Geometry: see drawing. Coordinates: mm, zero at the bounding-box minimum. A direction names the side the tool comes from. Coordinates: 2 decimals unless noted, no trailing zeros. Order: outer loops, then holes, each group sorted by start corner. A loop starts at its lowest first (then second) coordinate and runs counter-clockwise, first axis right, second up. Notation, with made-up numbers: M -21.5,-7 L 16.5,-7 A21 ccw 16.5,29 Z; hole C 3.5,51 d4. An arc over 180 degrees is marked long. Answer in a Markdown table with one row per item.
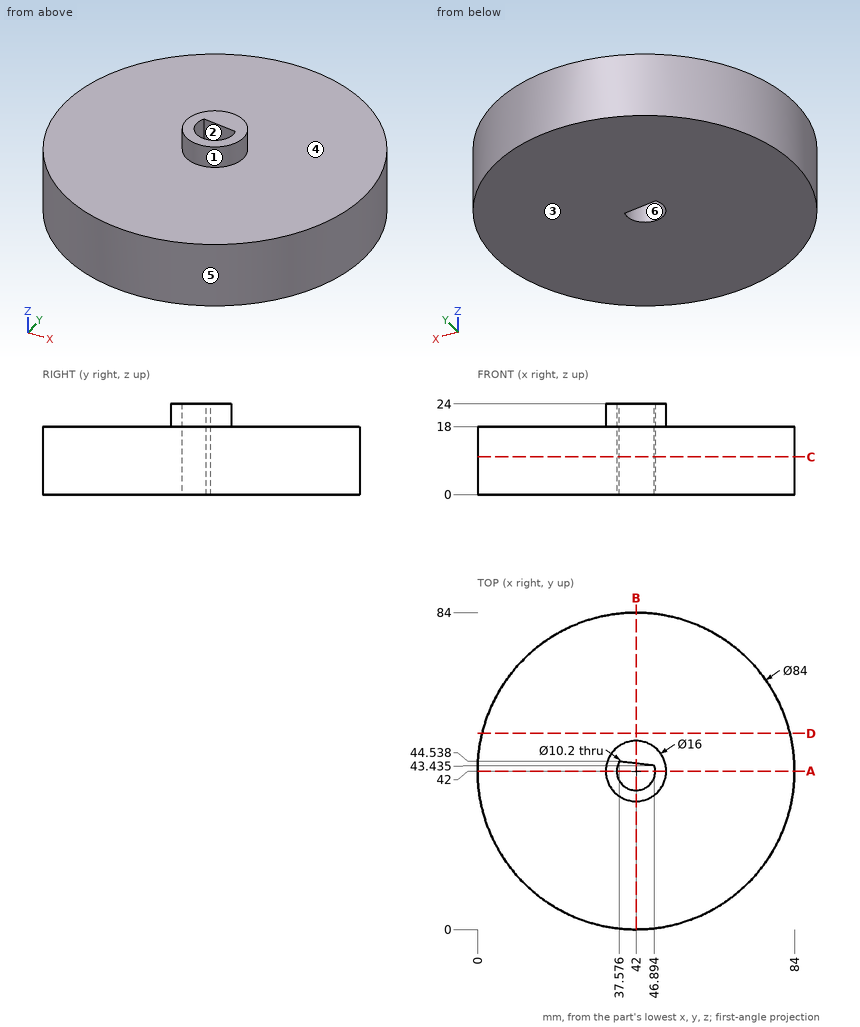
1) Cut plane D-D, the plane y = 52. Output: boundary loops of the cut face in (x, z).
Resolved:
| item | result |
|---|---|
| outline | M 1.21,0 L 82.79,0 L 82.79,18 L 1.21,18 Z |
2) Reachability of the marked faces 1, 2 and 3 from +Z, -Z, +X, -X, +Y, -Y: full face, straight path, thin tool, end or side. Return the list, or none.
Resolved:
| item | result |
|---|---|
| face 1 | +Z |
| face 2 | +Z, -Z |
| face 3 | -Z, +X, -X, +Y, -Y |
3) Contact query for flat-ended pins moving along their axis: pin 1 (5 mm diameter, centred on y = 17.5, z = 8.5, fed in from -X); pin 2 (3 mm diameter, centred on x = 30.5, y = 72.5, fed in from +Z); pin 3 (1.5 mm diameter, centred on x = 61, z = 20.5, fed in from +Y) (1 decimal); pin 4 (8 mm diameter, centred on y = 73, z = 13.5, fed in from -X). Output: stop coordinate, or through.
Resolved:
| item | result |
|---|---|
| pin 1 | stops at x = 6.22 |
| pin 2 | stops at z = 18 |
| pin 3 | passes through |
| pin 4 | stops at x = 9.83 |
4) Material intervals for probe 1 along X at (y, z) = (42, 15.25); probe 2 along Z at (x, y) = (15.5, 64); probe 3 along Y at (x, z) = (42, 12.5) (1 decimal), sorted ascending.
Resolved:
| item | result |
|---|---|
| probe 1 | x = 0 to 36.9, 47.1 to 84 |
| probe 2 | z = 0 to 18 |
| probe 3 | y = 0 to 36.9, 44 to 84 |
5) Cut plane A-A, the plane y = 42. Output: boundary loops of the cut face in (x, z).
Resolved:
| item | result |
|---|---|
| outline | M 0,0 L 36.9,0 L 36.9,24 L 34,24 L 34,18 L 0,18 Z; M 47.1,0 L 84,0 L 84,18 L 50,18 L 50,24 L 47.1,24 Z |
6) Mould query, pull axis Y, two halves, no side actions, for the marked faces 4, 5 and 6. Classes: +Y half, -Y half, draft (parallel to the pull), parting line (faces both ways), or undercut.
Resolved:
| item | result |
|---|---|
| face 4 | draft |
| face 5 | parting line |
| face 6 | undercut |
7) Cut plane C-C, the plane z = 10. Output: boundary loops of the cut face in (x, y) (1 decimal).
Resolved:
| item | result |
|---|---|
| outline | C 42,42 d84; hole M 37.6,44.5 A5.1 ccw long 46.9,43.4 Z |
8) Cut plane B-B, the plane x = 42. Output: boundary loops of the cut face in (y, z).
Resolved:
| item | result |
|---|---|
| outline | M 0,0 L 36.9,0 L 36.9,24 L 34,24 L 34,18 L 0,18 Z; M 44.01,0 L 84,0 L 84,18 L 50,18 L 50,24 L 44.01,24 Z |
